For this review, take the finished solid that the model builds, in its own axes (mm). A direction names the side the tool comes from. Coordinates: 2 decimals unless noted, no trailing zeros. Loops run counter-clockwise (first coordinate to the right, second up) from the corner with the lowest first, then second, coordinate; pieces in that order, holes last.
1. To check wall thickness, follow probe 1 along X at (y, z) = (-1, 21.5); probe 2 along X at (y, z) = (-3.75, 21); probe 3 along Y at (x, z) = (-27.5, 24.5). State the ranges of each line that lie inside material, in increasing order.
2. Clearance check with flat-ended pins moving along their axes: P1, Ø3, axis at x = 5.5, y = -1.5, coming from the +Z side; P2, Ø1.5, axis at y = -0.5, z = 22, coming from the -X side; P3, Ø4, axis at x = 7.5, z = 20.5, coming from the -Y side. State where each tip first meets the part, or that it passes through.
3. Take a section at C-C, the plane z = 24.25. State the section outline as (x, y) points, then the cut area to 3 significant figures.
4. Take a section at A-A, the plane y = -2.5. State the section outline as (x, z) points, then the cut area to 3 significant figures.
5. Machinability: for faces 1 (the face through (22.139, -1, 21)), 2 (the face through (26, -3, 18.537)), 3 (the face through (27, -3, 20.124)), which of the approach directions +Z, -Z, +X, -X, +Y, -Y give a long, thin tool a straight path to every point of the face, cutting with its end or side? Answer none if there is none.
6. Take a section at D-D, the plane x = 6.5. State the section outline as (y, z) points (3 decimals).
7. Mouldability with a two-part tool opening along Y and no side actions: class faces 4 (the face through (20.573, -4.457, 20.835)), 5 (the face through (32.346, -5.395, 19.342)), 6 (the face through (31.662, -3.105, 19.319)), 7 (the face through (23, 0, 24)) as pulls with the +Y half, pulls with the -Y half, needs draft (parallel to the pull), parting line crosses it, or undercut.
```python
from build123d import *

# Parameters (mm, degrees)
F1_DEPTH = 6.35
F2_R     = 3.17499
F4_D     = 3.175
F5_R     = 2.778125
F6_DEPTH = 3.175
F7_R     = 1.984375
F8_DEPTH = 52.3875


# Not quite as in the source:
# - a fillet or chamfer is up to 0.001 mm smaller than in the source, because OpenCascade refuses the exact size


with BuildPart() as f1:
    # F0 (on Front) → F1 (new body)
    with BuildSketch(Plane.XZ):
        Polygon((33.251190576, 26.4741850346), (33.251190576, 28.0616850346), (22.138690576, 28.0616850346), (22.138690576, 18.5366850346), (33.251190576, 18.5366850346), (33.251190576, 20.1241850346), (23.726190576, 20.1241850346), (23.726190576, 26.4741850346), align=None)
    extrude(amount=F1_DEPTH)

    # F2 (radius 3.175 in the source; OpenCascade refuses exactly that, so slightly less here)
    f2_edges = [f1.edges().sort_by_distance(p)[0] for p in [
        (33.251191, -6.35, 19.330435),
        (33.251191, -6.35, 27.267935),
        (33.251191, 0, 27.267935),
        (33.251191, 0, 19.330435),
    ]]
    fillet(f2_edges, radius=F2_R)

    # F4 (through all)
    with Locations(Plane.XY.offset(28.0616850346)):
        with Locations((30.076190576, -3.175)):
            Hole(F4_D / 2)

    # F5 (on face) → F6 (join)
    with BuildSketch(Plane(origin=(22.138690576, 0, 0), x_dir=(0, -1, 0), z_dir=(-1, 0, 0))):
        with Locations((3.175, 23.2991850346)):
            Circle(F5_R)
    extrude(amount=F6_DEPTH)

    # F7 (on face) → F8 (join)
    with BuildSketch(Plane(origin=(18.963690576, 0, 0), x_dir=(0, -1, 0), z_dir=(-1, 0, 0))):
        with Locations((3.175, 23.2991850346)):
            Circle(F7_R)
    extrude(amount=F8_DEPTH)


solid = f1.part
```
Results list:
1. probe 1: x = 22.14 to 23.73
1. probe 2: x = 18.96 to 23.73
1. probe 3: y = -4.75 to -1.6
2. P1: stops at z = 25.28
2. P2: stops at x = 18.96
2. P3: stops at y = -4.99
3. outline: (-33.42, -4.92) - (18.96, -4.92) - (18.96, -5.79) - (22.14, -5.79) - (22.14, -6.35) - (23.73, -6.35) - (23.73, 0) - (22.14, 0) - (22.14, -0.56) - (18.96, -0.56) - (18.96, -1.43) - (-33.42, -1.43) - close
3. area: 209 mm2
4. outline: (-33.42, 21.43) - (18.96, 21.43) - (18.96, 20.6) - (22.14, 20.6) - (22.14, 18.54) - (28.64, 18.54) - (28.64, 20.12) - (23.73, 20.12) - (23.73, 26.47) - (28.64, 26.47) - (28.64, 28.06) - (22.14, 28.06) - (22.14, 25.99) - (18.96, 25.99) - (18.96, 25.17) - (-33.42, 25.17) - close; (31.51, 18.54) - (33.18, 18.54) - (33.18, 20.12) - (31.51, 20.12) - close; (31.51, 26.47) - (33.18, 26.47) - (33.18, 28.06) - (31.51, 28.06) - close
4. area: 249 mm2
5. face 1: -X
5. face 2: -Z, +X, -X, +Y, -Y
5. face 3: +X, +Y, -Y
6. outline: circle Ø3.969 at (-3.175, 23.299)
7. face 4: parting line crosses it
7. face 5: pulls with the -Y half
7. face 6: undercut
7. face 7: pulls with the +Y half
